The listing builds one solid part. Answer for the finished solid, in the listing's coordinates (mm). Give positions to 0.01 mm unless a question says otherwise; leave off trailing zeros. Write each loop counter-clockwise with the first axis right and the second up, starting at its lowest first coordinate (ties: lowest second). Pieces come first, ordered by that corner, then holes. Notation, with made-up numbers: (47, -18) - (83, -18) arc R11 ccw to (83, 2) - close; hole circle Ø8 at (-1.75, 14). An arc over 180 degrees is marked (long way). Answer as CSV lines item,"result". Start each with the question number.
(1) Find section A-A (x = 35.56). Write down the section's boundary in (y, z).
(2) Straight lines are drawn through the part: probe 1 along Y at (x, z) = (35.56, 0.95); probe 2 along Y at (x, z) = (35, 2.5); probe 3 along X at (y, z) = (5.5, 1.45). For each, find the intervals that lie inside material, in ascending order.
(3) Find section B-B (z = 1.5). Write down the section's boundary in (x, y) (1 decimal).
(4) This flat-tipped pin is pushed along its axis until it touches: pin 1 Ø3 at (x, y) = (68.45, 3.11) entering from -Z. Where does it stop, or does it pass through?
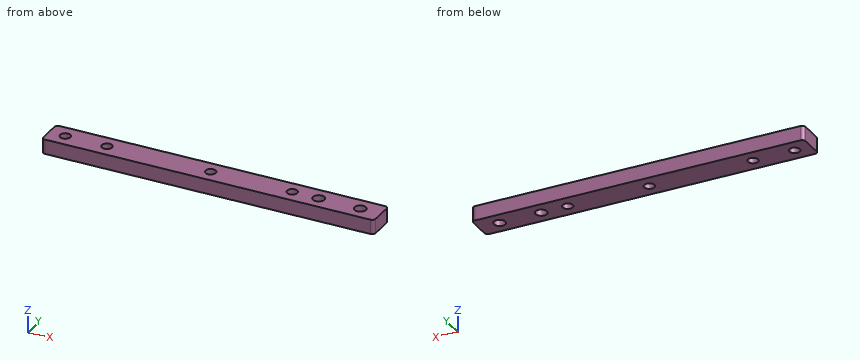
from build123d import *

# Parameters (mm, degrees)
SKETCH1_W           = 73.025
SKETCH1_H           = 6.223
SKETCH1_R           = 1.27
SKETCH1_R_2         = 1.1303
BOSS_EXTRUDE1_DEPTH = 3.2004
SKETCH2_R           = 1.1303
CUT_EXTRUDE1_DEPTH  = 3.2004
FILLET1_R           = 0.762


with BuildPart() as part:
    # Sketch1 → Boss-Extrude1 (new body)
    with BuildSketch(Plane.XY):
        with Locations((36.5125, 3.1115)):
            Rectangle(SKETCH1_W, SKETCH1_H)
        with Locations((59.309, 3.1115)):
            Circle(SKETCH1_R, mode=Mode.SUBTRACT)
        with Locations((68.453, 3.1115)):
            Circle(SKETCH1_R, mode=Mode.SUBTRACT)
        with Locations((3.6195, 3.1115)):
            Circle(SKETCH1_R_2, mode=Mode.SUBTRACT)
        with Locations((12.7635, 3.1115)):
            Circle(SKETCH1_R_2, mode=Mode.SUBTRACT)
    extrude(amount=BOSS_EXTRUDE1_DEPTH)

    # Sketch2 → Cut-Extrude1 (cut)
    with BuildSketch(Plane.XY.offset(3.2004)):
        with Locations((35.56, 3.1115)):
            Circle(SKETCH2_R)
        with Locations((53.4924, 3.1115)):
            Circle(SKETCH2_R)
    extrude(amount=-CUT_EXTRUDE1_DEPTH, mode=Mode.SUBTRACT)

    # Fillet1
    fillet1_edges = [part.edges().sort_by_distance(p)[0] for p in [
        (0, 6.223, 1.6002),
        (73.025, 6.223, 1.6002),
        (73.025, 0, 1.6002),
        (0, 0, 1.6002),
    ]]
    fillet(fillet1_edges, radius=FILLET1_R)


solid = part.part
Result set:
1,outline,"(0, 0) - (1.98, 0) - (1.98, 3.2) - (0, 3.2) - close; (4.24, 0) - (6.22, 0) - (6.22, 3.2) - (4.24, 3.2) - close"
2,probe 1,"0 to 1.98, 4.24 to 6.22"
2,probe 2,"0 to 2.13, 4.09 to 6.22"
2,probe 3,"0 to 73.02"
3,outline,"(0, 0.8) arc R0.8 ccw to (0.8, 0) - (72.3, 0) arc R0.8 ccw to (73, 0.8) - (73, 5.5) arc R0.8 ccw to (72.3, 6.2) - (0.8, 6.2) arc R0.8 ccw to (0, 5.5) - close; hole circle Ø2.3 at (3.6, 3.1); hole circle Ø2.3 at (12.8, 3.1); hole circle Ø2.3 at (35.6, 3.1); hole circle Ø2.3 at (53.5, 3.1); hole circle Ø2.5 at (59.3, 3.1); hole circle Ø2.5 at (68.5, 3.1)"
4,pin 1,"z = 0"
